Autodesk Inventor part; units mm, degrees
sketch "Sketch1" plane through (0, 0, 0) normal (0, 0, 1) x (1, 0, 0)
  circle A0 centre (0, 0) radius 40.7
  dimension "d0" = 81.4
extrude "Extrusion1" add sketch "Sketch1" along normal blind 21.75
sketch "Sketch2" plane through (0, 0, 21.75) normal (0, 0, 1) x (1, 0, 0)
  circle A0 centre (0, 0) radius 22
  dimension "d3" = 44
extrude "Extrusion2" cut sketch "Sketch2" against normal blind 9
sketch "Sketch3" plane through (0, 0, 12.75) normal (0, 0, 1) x (1, 0, 0)
  circle A0 centre (0, 18) radius 2
  circle A1 centre (-18, 0) radius 2
  circle A2 centre (0, -18) radius 2
  circle A3 centre (18, 0) radius 2
  point P0 (0, 0)
  dimension "d6" = 4
  dimension "d7" = 18
  dimension "d10" = 360
extrude "Extrusion3" cut sketch "Sketch3" against normal blind 12.75
sketch "Sketch4" plane through (0, 0, 12.75) normal (0, 0, 1) x (1, 0, 0)
  arc A0 (-4.5165, 17.448) -> (-8.8542, 19.2414) centre (-7.5165, 16.3345) ccw
  arc A1 (-8.8542, 19.2414) -> (-19.0977, 9.16) centre (0, 0) ccw
  arc A2 (-14.1333, 4.5) -> (-11.4833, 6.0938) centre (-14.1333, 7.5) ccw
  line L0 (-4.5, 14.1333) -> (-4.5, 16.3631)
  arc A3 (-4.5, 16.3631) -> (-8.75, 19.0902) centre (-7.5, 16.3631) ccw
  arc A4 (-6.0938, 11.4833) -> (-4.5, 14.1333) centre (-7.5, 14.1333) ccw
  arc A5 (-6.0938, 11.4833) -> (-11.4833, 6.0938) centre (0, 0) ccw
  arc A6 (-8.8542, 19.2414) -> (-19.2547, 8.8254) centre (0, 0) ccw
  arc A7 (-8.75, 19.0902) -> (-19.0902, 8.75) centre (0, 0) ccw
  arc A8 (-19.0902, 8.75) -> (-16.3631, 4.5) centre (-16.3631, 7.5) ccw
  line L1 (-16.3631, 4.5) -> (-14.1333, 4.5)
  arc A9 (-11.4833, -6.0938) -> (-14.1333, -4.5) centre (-14.1333, -7.5) ccw
  arc A10 (-4.5, -14.1333) -> (-6.0938, -11.4833) centre (-7.5, -14.1333) ccw
  arc A11 (-11.4833, -6.0938) -> (-6.0938, -11.4833) centre (0, 0) ccw
  line L2 (-14.1333, -4.5) -> (-16.3631, -4.5)
  line L3 (-4.5, -16.3631) -> (-4.5, -14.1333)
  arc A12 (-16.3631, -4.5) -> (-19.0902, -8.75) centre (-16.3631, -7.5) ccw
  arc A13 (-17.448, -4.5165) -> (-19.2414, -8.8542) centre (-16.3345, -7.5165) ccw
  arc A14 (-8.75, -19.0902) -> (-4.5, -16.3631) centre (-7.5, -16.3631) ccw
  arc A15 (-19.0902, -8.75) -> (-8.75, -19.0902) centre (0, 0) ccw
  arc A16 (-19.2414, -8.8542) -> (-9.16, -19.0977) centre (0, 0) ccw
  arc A17 (-19.2414, -8.8542) -> (-8.8254, -19.2547) centre (0, 0) ccw
  arc A18 (6.0938, -11.4833) -> (4.5, -14.1333) centre (7.5, -14.1333) ccw
  arc A19 (14.1333, -4.5) -> (11.4833, -6.0938) centre (14.1333, -7.5) ccw
  arc A20 (6.0938, -11.4833) -> (11.4833, -6.0938) centre (0, 0) ccw
  line L4 (4.5, -14.1333) -> (4.5, -16.3631)
  line L5 (16.3631, -4.5) -> (14.1333, -4.5)
  arc A21 (4.5, -16.3631) -> (8.75, -19.0902) centre (7.5, -16.3631) ccw
  arc A22 (4.5165, -17.448) -> (8.8542, -19.2414) centre (7.5165, -16.3345) ccw
  arc A23 (19.0902, -8.75) -> (16.3631, -4.5) centre (16.3631, -7.5) ccw
  arc A24 (8.75, -19.0902) -> (19.0902, -8.75) centre (0, 0) ccw
  arc A25 (8.8542, -19.2414) -> (19.0977, -9.16) centre (0, 0) ccw
  arc A26 (8.8542, -19.2414) -> (19.2547, -8.8254) centre (0, 0) ccw
  arc A27 (11.4833, 6.0938) -> (14.1333, 4.5) centre (14.1333, 7.5) ccw
  arc A28 (4.5, 14.1333) -> (6.0938, 11.4833) centre (7.5, 14.1333) ccw
  arc A29 (11.4833, 6.0938) -> (6.0938, 11.4833) centre (0, 0) ccw
  line L6 (14.1333, 4.5) -> (16.3631, 4.5)
  line L7 (4.5, 16.3631) -> (4.5, 14.1333)
  arc A30 (16.3631, 4.5) -> (19.0902, 8.75) centre (16.3631, 7.5) ccw
  arc A31 (17.448, 4.5165) -> (19.2414, 8.8542) centre (16.3345, 7.5165) ccw
  arc A32 (8.75, 19.0902) -> (4.5, 16.3631) centre (7.5, 16.3631) ccw
  arc A33 (19.0902, 8.75) -> (8.75, 19.0902) centre (0, 0) ccw
  arc A34 (19.2414, 8.8542) -> (9.16, 19.0977) centre (0, 0) ccw
  arc A35 (19.2414, 8.8542) -> (8.8254, 19.2547) centre (0, 0) ccw
  point P0 (41.0732, 32.7294)
  point P1 (-17.4931, 4.4714)
  point P2 (-16.3796, 7.4714)
  point P3 (-7.4714, -16.3796)
  point P4 (-4.4714, -17.4931)
  point P5 (16.3796, -7.4714)
  point P6 (17.4931, -4.4714)
  point P7 (7.4714, 16.3796)
  point P8 (4.4714, 17.4931)
  dimension "d16" = 360
extrude "Extrusion4" cut sketch "Sketch4" against normal blind 12.75
ref_plane "Work Plane1" through (40.7, 0, 0) normal (1, 0, 0) x (0, 1, 0)
properties part number "MotorHousing" material "Plastic, Opaque White"
Input: part model. Units: mm. Frame: model coordinates. Give positions to 0.01 mm unless a question says otherwise; leave off trailing zeros. Order: outer loops, then holes, each group sorted by start corner. A loop starts at its lowest first (then second) coordinate and runs counter-clockwise, first axis right, second up. Notation, with made-up numbers: M -5,15 L 40,15 A22 ccw 40,50 Z; hole C 40.5,33.25 d9. An arc over 180 degrees is marked long. Return JSON: item names as keys, results as strings.
1) Line query: L1, parallel to X at y = 13, z = 7.5; L2, parallel to X at y = -13.5, z = 1.5; L3, parallel to Y at x = 0, z = 6. Output: solid intervals per line, ascending. Write a range as [from, to].
Taken from the geometry:
{"L1": "x = [-38.57, -16.49], [-4.72, 4.72], [16.49, 38.57]", "L2": "x = [-38.4, -16.09], [-4.57, 4.57], [16.09, 38.4]", "L3": "y = [-40.7, -20], [-16, 16], [20, 40.7]"}
2) Contact query for flat-ended pins moving along their axis: pin 1 (4.5 mm diameter, centred on x = 0, y = 18, fed in from +Z); pin 2 (2.5 mm diameter, centred on y = -15, z = 5, fed in from +X); pin 3 (2.5 mm diameter, centred on x = 15, z = 7, fed in from -Y); pin 4 (3 mm diameter, centred on x = -18, y = 0, fed in from +Z). Output: stop coordinate, or through.
Taken from the geometry:
{"pin 1": "stops at z = 12.75", "pin 2": "stops at x = 38.31", "pin 3": "stops at y = -38.31", "pin 4": "passes through"}
3) Section query A-A on x = 0. Output: boundary loops of the cut face in (y, z).
Taken from the geometry:
{"outline": "M -40.7,0 L -20,0 L -20,12.75 L -22,12.75 L -22,21.75 L -40.7,21.75 Z; M -16,0 L 16,0 L 16,12.75 L -16,12.75 Z; M 20,0 L 40.7,0 L 40.7,21.75 L 22,21.75 L 22,12.75 L 20,12.75 Z"}
4) Mould query, pull axis X, two halves, no side actions, for faces 1 (the face through (5.9, 18.9, 6.5)), 2 (the face through (18, -18, 21.75)). Classes: released by +X, released by -X, zero draft, split by the parting line, or undercut.
Taken from the geometry:
{"face 1": "undercut", "face 2": "zero draft"}
5) Section query C-C on y = -18. Output: boundary loops of the cut face in (x, z).
Taken from the geometry:
{"outline": "M -36.5,0 L -10.82,0 L -10.82,12.75 L -12.65,12.75 L -12.65,21.75 L -36.5,21.75 Z; M -4.99,0 L -2,0 L -2,12.75 L -4.99,12.75 Z; M 2,0 L 4.99,0 L 4.99,12.75 L 2,12.75 Z; M 10.82,0 L 36.5,0 L 36.5,21.75 L 12.65,21.75 L 12.65,12.75 L 10.82,12.75 Z"}
